Design review of the part built by this model. Coordinates are the model's own, in mm. Face numbers are marked on the shaded views. A direction names the side the tool comes from. Coordinates: 2 decimals unless noted, no trailing zeros. Loops run counter-clockwise (first coordinate to the right, second up) from the corner with the lowest first, then second, coordinate; pieces in that order, holes last. Notation, with made-up numbers: M 55.5,0 L 93.5,0 A22 ccw 93.5,13 Z; hole C 7,-25.5 d10. An arc over 180 degrees is marked long. Answer as a JSON object with one key per item and string values. Group by question number.
1. Consider section A-A (z = -18.25). State the section outline as (x, y) points (3 decimals), then the cut area to 3 significant figures.
2. Consider section D-D (x = -11.25). State the section outline as (y, z) points (3 decimals), then the cut area to 3 significant figures.
3. To check wall thickness, follow probe 1 along Y at (x, z) = (-24.45, -12.7) (3 decimals); probe 2 along Z at (x, y) = (-11.75, 45.5) (3 decimals); probe 3 along Y at (x, z) = (-1, -14.75). State the ranges of each line that lie inside material, in increasing order.
4. Consider section B-B (y = 38.1). State the section outline as (x, z) points (3 decimals).
5. Machinability: for the marked faces 1 and 2, which of the approach directions +Z, -Z, +X, -X, +Y, -Y give a long, thin tool a straight path to every point of the face, cutting with its end or side? Answer none if there is none.
6. Consider section C-C (z = -12.7). State the section outline as (x, y) points (3 decimals).
7. Draft analysis for pull direction X (two halves, no side actions). For the marked faces 3, 4, 5 and 6, state which applies: +X half, -X half, draft (parallel to the pull), parting line (faces both ways), or undercut.
Autodesk Inventor part; units mm, degrees
ref_plane "YZ Plane" through (0, 0, 0) normal (1, 0, 0) x (0, 1, 0)
ref_plane "XZ Plane" through (0, 0, 0) normal (0, 1, 0) x (-1, 0, 0)
ref_plane "XY Plane" through (0, 0, 0) normal (0, 0, 1) x (1, 0, 0)
sketch "Sketch1" plane through (0, 0, 0) normal (0, 1, 0) x (-1, 0, 0)
  line L0 (0, 0) -> (25.4, 0)
  line L1 (25.4, 0) -> (25.4, -25.4)
  line L2 (25.4, -25.4) -> (0, -25.4)
  line L3 (0, -25.4) -> (0, 0)
  line L4 (22.225, -22.225) -> (22.225, -3.175)
  line L5 (22.225, -3.175) -> (3.175, -3.175)
  line L6 (3.175, -3.175) -> (3.175, -22.225)
  line L7 (3.175, -22.225) -> (22.225, -22.225)
  dimension "d0" = 25.4
  dimension "d1" = 25.4
  dimension "d2" = 3.175
extrude "Extrusion1" add sketch "Sketch1" along normal blind 50.8
sketch "Sketch2" plane through (0, 0, 0) normal (1, 0, 0) x (0, 0, -1)
  line L0 (25.4, 0) -> (0, 0)
  line L1 (25.4, 0) -> (25.4, 50.8)
  line L2 (0, 50.8) -> (25.4, 50.8)
  line L3 (0, 0) -> (0, 50.8)
  point P0 (12.7, 38.1)
  point P1 (12.7, 12.7)
  dimension "d5" = 12.7
  dimension "d6" = 12.7
  dimension "d7" = 12.7
  dimension "d8" = 12.7
hole "Hole1" at (0, 38.1, -12.7) at (0, 12.7, -12.7) direction (-1, 0, 0) diameter 6.35 end through all
properties part number "1x1AluminumStandoff.ver1-1111-2020"
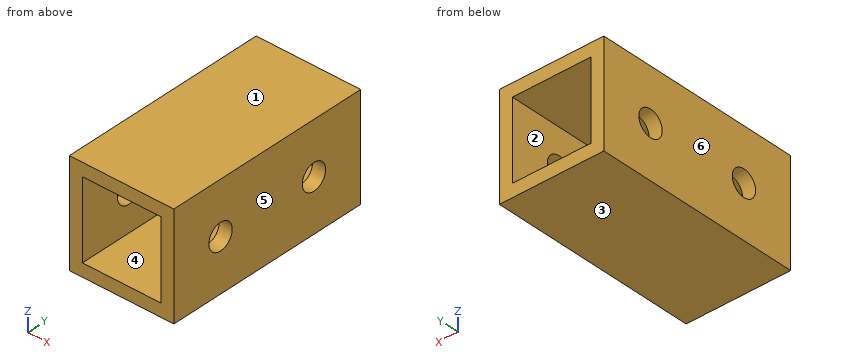
Findings below:
{
 "1": {"outline": "M -25.4,0 L -22.225,0 L -22.225,50.8 L -25.4,50.8 Z; M -3.175,0 L 0,0 L 0,50.8 L -3.175,50.8 Z", "area": "323 mm^2"},
 "2": {"outline": "M 0,-25.4 L 50.8,-25.4 L 50.8,-22.225 L 0,-22.225 Z; M 0,-3.175 L 50.8,-3.175 L 50.8,0 L 0,0 Z", "area": "323 mm^2"},
 "3": {"probe 1": "y = 0 to 9.525, 15.875 to 34.925, 41.275 to 50.8", "probe 2": "z = -25.4 to -22.225, -3.175 to 0", "probe 3": "y = 0 to 10.28, 15.12 to 35.68, 40.52 to 50.8"},
 "4": {"outline": "M -25.4,-25.4 L 0,-25.4 L 0,-15.875 L -3.175,-15.875 L -3.175,-22.225 L -22.225,-22.225 L -22.225,-15.875 L -25.4,-15.875 Z; M -25.4,-9.525 L -22.225,-9.525 L -22.225,-3.175 L -3.175,-3.175 L -3.175,-9.525 L 0,-9.525 L 0,0 L -25.4,0 Z"},
 "5": {"face 1": "+Z, +X, -X, +Y, -Y", "face 2": "+Y, -Y"},
 "6": {"outline": "M -25.4,0 L -22.225,0 L -22.225,9.525 L -25.4,9.525 Z; M -25.4,15.875 L -22.225,15.875 L -22.225,34.925 L -25.4,34.925 Z; M -25.4,41.275 L -22.225,41.275 L -22.225,50.8 L -25.4,50.8 Z; M -3.175,0 L 0,0 L 0,9.525 L -3.175,9.525 Z; M -3.175,15.875 L 0,15.875 L 0,34.925 L -3.175,34.925 Z; M -3.175,41.275 L 0,41.275 L 0,50.8 L -3.175,50.8 Z"},
 "7": {"face 3": "draft", "face 4": "undercut", "face 5": "+X half", "face 6": "-X half"}
}
